from build123d import *

# Parameters (mm, degrees)
BOSS_EXTRUDE1_DEPTH = 1.8
SKETCH2_W           = 69
SKETCH2_H           = 21
SKETCH2_W_2         = 65
SKETCH2_H_2         = 17
BOSS_EXTRUDE2_DEPTH = 15
SKETCH3_W           = 2
SKETCH3_H           = 14.5
CUT_EXTRUDE2_DEPTH  = 15
SKETCH4_W           = 69
SKETCH4_H           = 10.4
CUT_EXTRUDE4_DEPTH  = 13
BOSS_EXTRUDE4_DEPTH = 15
SKETCH8_W           = 16
SKETCH8_H           = 8.6
BOSS_EXTRUDE5_DEPTH = 10
SKETCH9_R           = 2.5
CUT_EXTRUDE5_DEPTH  = 12
CUT_EXTRUDE6_DEPTH  = 4
FILLET1_R           = 1.4
SKETCH11_W          = 8.5
SKETCH11_H          = 4.75
CUT_EXTRUDE7_DEPTH  = 4
FILLET2_R           = 1.4
FILLET6_R           = 1.5
FILLET7_R           = 1.5
FILLET8_R           = 3
FILLET9_R           = 1


with BuildPart() as part:
    # Sketch1 → Boss-Extrude1 (new body)
    with BuildSketch(Plane.XY):
        Polygon((0, 0), (72, 0), (72, 22.5), (73.5, 22.5), (73.5, 24), (72, 24), (0, 24), (-1.5, 24), (-1.5, 22.5), (0, 22.5), align=None)
    extrude(amount=BOSS_EXTRUDE1_DEPTH)

    # Sketch2 → Boss-Extrude2 (add)
    with BuildSketch(Plane(origin=(0, 0, 0), x_dir=(-1, 0, 0), z_dir=(0, 0, -1))):
        with Locations((-36, 12)):
            Rectangle(SKETCH2_W, SKETCH2_H)
        with Locations((-36, 12)):
            Rectangle(SKETCH2_W_2, SKETCH2_H_2, mode=Mode.SUBTRACT)
    extrude(amount=BOSS_EXTRUDE2_DEPTH)

    # Sketch3 → Cut-Extrude2 (cut)
    with BuildSketch(Plane(origin=(0, 0, -15), x_dir=(-1, 0, 0), z_dir=(0, 0, -1))):
        with Locations((-2.5, 13.25)):
            Rectangle(SKETCH3_W, SKETCH3_H)
    extrude(amount=-CUT_EXTRUDE2_DEPTH, mode=Mode.SUBTRACT)

    # Sketch4 → Cut-Extrude4 (cut)
    with BuildSketch(Plane(origin=(0, 0, -15), x_dir=(-1, 0, 0), z_dir=(0, 0, -1))):
        with Locations((-36, 17.3)):
            Rectangle(SKETCH4_W, SKETCH4_H)
    extrude(amount=-CUT_EXTRUDE4_DEPTH, mode=Mode.SUBTRACT)

    # Sketch7 → Boss-Extrude4 (add)
    with BuildSketch(Plane(origin=(0, 0, -15), x_dir=(-1, 0, 0), z_dir=(0, 0, -1))):
        Polygon((-68.5, 12.1), (-61.151923341, 12.1), (-61.151923341, 10.5), (-61.151923341, 3.5), (-62.751923341, 3.5), (-62.751923341, 10.5), (-68.5, 10.5), align=None)
    extrude(amount=-BOSS_EXTRUDE4_DEPTH)

    # Sketch8 → Boss-Extrude5 (add)
    with BuildSketch(Plane(origin=(0, 0, 0), x_dir=(-1, 0, 0), z_dir=(0, 0, -1))):
        with Locations((-53.151923341, 7.8)):
            Rectangle(SKETCH8_W, SKETCH8_H)
    extrude(amount=BOSS_EXTRUDE5_DEPTH)

    # Sketch9 → Cut-Extrude5 (cut)
    with BuildSketch(Plane(origin=(0, 0, -10), x_dir=(-1, 0, 0), z_dir=(0, 0, -1))):
        with Locations((-49.651923341, 7.8)):
            Circle(SKETCH9_R)
        with Locations((-57.651923341, 7.8)):
            Circle(SKETCH9_R)
    extrude(amount=-CUT_EXTRUDE5_DEPTH, mode=Mode.SUBTRACT)

    # Sketch10 → Cut-Extrude6 (cut)
    with BuildSketch(Plane(origin=(0, 0, -10), x_dir=(-1, 0, 0), z_dir=(0, 0, -1))):
        with BuildLine():
            Line((-57.651923341, 11.3), (-49.651923341, 11.3))
            ThreePointArc((-49.651923341, 11.3), (-46.151923341, 7.8), (-49.651923341, 4.3))
            Line((-49.651923341, 4.3), (-57.651923341, 4.3))
            ThreePointArc((-57.651923341, 4.3), (-61.151923341, 7.8), (-57.651923341, 11.3))
        make_face()
    extrude(amount=-CUT_EXTRUDE6_DEPTH, mode=Mode.SUBTRACT)

    # Fillet1
    fillet1_edges = [part.edges().sort_by_distance(p)[0] for p in [
        (52.151923341, 7.8, 1.8),
        (60.151923341, 7.8, 1.8),
    ]]
    fillet(fillet1_edges, radius=FILLET1_R)

    # Sketch11 → Cut-Extrude7 (cut)
    with BuildSketch(Plane.XY.offset(1.8)):
        with Locations((14, 6.125)):
            Rectangle(SKETCH11_W, SKETCH11_H)
    extrude(amount=-CUT_EXTRUDE7_DEPTH, mode=Mode.SUBTRACT)

    # Fillet2
    fillet2_edges = [part.edges().sort_by_distance(p)[0] for p in [
        (9.75, 6.125, 1.8),
        (14, 3.75, 1.8),
        (18.25, 6.125, 1.8),
        (14, 8.5, 1.8),
    ]]
    fillet(fillet2_edges, radius=FILLET2_R)

    # Fillet6
    fillet6_edges = [part.edges().sort_by_distance(p)[0] for p in [
        (70.5, 1.5, -7.5),
        (1.5, 1.5, -7.5),
    ]]
    fillet(fillet6_edges, radius=FILLET6_R)

    # Fillet7
    fillet7_edges = [part.edges().sort_by_distance(p)[0] for p in [
        (70.5, 22.5, -1),
        (1.5, 22.5, -1),
    ]]
    fillet(fillet7_edges, radius=FILLET7_R)

    # Fillet8
    fillet8_edges = [part.edges().sort_by_distance(p)[0] for p in [
        (72, 0, 0.9),
        (0, 0, 0.9),
    ]]
    fillet(fillet8_edges, radius=FILLET8_R)

    # Fillet9
    fillet9_edges = [part.edges().sort_by_distance(p)[0] for p in [
        (72, 12.75, 1.8),
        (36, 0, 1.8),
        (0.878679656, 0.878679656, 1.8),
        (71.121320344, 0.878679656, 1.8),
        (0, 12.75, 1.8),
    ]]
    fillet(fillet9_edges, radius=FILLET9_R)


solid = part.part
The listing builds one solid part. Answer for the finished solid, in the listing's coordinates (mm). A direction names the side the tool comes from. Coordinates: 2 decimals unless noted, no trailing zeros. Loops run counter-clockwise (first coordinate to the right, second up) from the corner with the lowest first, then second, coordinate; pieces in that order, holes last.
1) Find section D-D on x = 21.5. Write down the section's boundary in (y, z), then the cut area to 3 significant figures.
2) Find section B-B on y = 15. Write down the section's boundary in (x, z).
3) Flat-ended cylindrical pins translate along their axes: pin 1 Ø4 at (x, z) = (27.5, -8.5) entering from +Y; pin 2 Ø4.5 at (y, z) = (14.5, -4) entering from +X; pin 3 Ø1.5 at (y, z) = (21.5, 0) entering from +X. Find the tip coordinate at first contact, or state that the pin passes through.
4) Find section C-C on z = -4. Write down the section's boundary in (x, y).
5) Find section A-A on z = -9.25. Write down the section's boundary in (x, y), then the cut area to 3 significant figures.
6) A tool of negligible diameter and unlimited length cuts with its end or side. For faces 5 (the face through (36, 1.5, -7)), 6 (the face through (36, 22.5, -1)), 7 (the face through (18.86, 6.178, 1.556)), 8 (the face through (58, 12.1, -6)), 9 (the face through (1.5, 4, -7)), from which of +Z, -Z, +X, -X, +Y, -Y can it reach the whole face along a straight path? Write none if from no direction.
7) Determine the mould class of faces 1 (the face through (54, 11.3, -8)), 2 (the face through (35, 13, 1.8)), 3 (the face through (68.5, 7, -7)), 4 (the face through (70.5, 8, -7)) for opening direction X: pulls with the +X half, pulls with the -X half, needs draft (parallel to the pull), parting line crosses it, or undercut.
8) Find the intervals of material crossed by L1, parallel to X at y = 8.75, z = -11.75; L2, parallel to Y at x = 68, z = -1.5; L3, parallel to X at y = 9.5, z = 0.5, in increasing order.
Values:
1. outline: (0, 0) - (1.5, 0) - (1.5, -15) - (3.5, -15) - (3.5, 0) - (20.5, 0) - (20.5, -2) - (22.5, -2) - (22.5, 0) - (24, 0) - (24, 1.8) - (1, 1.8) arc R1 ccw to (0, 0.8) - close
1. area: 77.0 mm2
2. outline: (0, 0) - (68.5, 0) - (68.5, -2) - (70.5, -2) - (70.5, 0) - (72, 0) - (72, 0.8) arc R1 ccw to (71, 1.8) - (1, 1.8) arc R1 ccw to (0, 0.8) - close
3. pin 1: stops at y = 3.5
3. pin 2: stops at x = 70.5
3. pin 3: stops at x = 72
4. outline: (1.5, 3) arc R1.5 ccw to (3, 1.5) - (69, 1.5) arc R1.5 ccw to (70.5, 3) - (70.5, 12.1) - (45.15, 12.1) - (45.15, 3.5) - (3.5, 3.5) - (3.5, 6) - (1.5, 6) - close; hole circle Ø5 at (49.65, 7.8); hole circle Ø5 at (57.65, 7.8); hole (62.75, 3.5) - (68.5, 3.5) - (68.5, 10.5) - (62.75, 10.5) - close
5. outline: (1.5, 3) arc R1.5 ccw to (3, 1.5) - (69, 1.5) arc R1.5 ccw to (70.5, 3) - (70.5, 12.1) - (45.15, 12.1) - (45.15, 3.5) - (3.5, 3.5) - (3.5, 6) - (1.5, 6) - close; hole (49.65, 4.3) - (57.65, 4.3) arc R3.5 ccw to (57.65, 11.3) - (49.65, 11.3) arc R3.5 ccw to start; hole (62.75, 3.5) - (68.5, 3.5) - (68.5, 10.5) - (62.75, 10.5) - close
5. area: 225 mm2
6. face 5: -Z, +X, -X, -Y
6. face 6: -Z, +X, -X, +Y
6. face 7: +Z
6. face 8: -Z, -X
6. face 9: -Z, -X, +Y, -Y
7. face 1: undercut
7. face 2: needs draft
7. face 3: undercut
7. face 4: pulls with the +X half
8. L1: x = 61.15 to 62.75, 68.5 to 70.5
8. L2: y = 1.5 to 3.5, 10.5 to 12.1, 20.5 to 22.5
8. L3: x = 0 to 47.81, 51.49 to 55.81, 59.49 to 72
